Can you work these out from the model? Positions are in its coordinate system, mm. Face numbers are marked on the shaded views. A direction names the side the tool comes from. Coordinates: 2 decimals unless noted, no trailing zeros. Order: outer loops, then holes, each group sorted by start corner. A loop starts at its lowest first (then second) coordinate and runs counter-clockwise, first axis right, second up. Notation, with made-up numbers: (-36.5, 25) -> (13.5, 25) arc R36 cw to (13.5, 59) -> close; hole circle Ø1 at (12, -11). An arc over 180 degrees is marked (long way). Use a Markdown table: item, result. Add a question column.
1. If I drill on line 1 along Z through (x, y) = (-25, -5.25); line 2 along Y through (x, z) = (-4.5, 2); line 3 along X through (y, z) = (-3.25, -3.5), over which ranges is the centre line in solid material (lowest first)? Write a range as from..to.
2. Suppose I cut it at C-C, the plane y = -1.75. List the corners of the cut face in (x, z) for me, then the cut area to 3 significant figures.
3. Suppose I cut it at A-A, the plane x = -24. List the corners of the cut face in (y, z) for me, then the cut area to 3 significant figures.
4. For pin 1 Ø14 at (x, z) = (-13, -1) entering from -Y; pin 2 Ø8 at (y, z) = (-3, -1.5) entering from -X; pin 3 Ø4 at (x, z) = (-21.5, -5) entering from +Y, each with a flat end and sliding along its axis, tell me the tip position at first contact or that it passes through.
5. Suppose I cut it at B-B, the plane x = -5. List the corners of the cut face in (y, z) for me.
6. Suppose I cut it at D-D, the plane z = 14.5. List the corners of the cut face in (x, y) for me.
7. We'd pull the mould along Z, two halves only. Please class the marked faces 4, 5, 6 and 7: pulls with the +Z half, pulls with the -Z half, needs draft (parallel to the pull), parting line crosses it, or undercut.
8. For the marked faces 1, 2 and 3, which set-ups out of +Z, -Z, +X, -X, +Y, -Y let a thin tool reach every point of the face, with its end or its side?
```python
from build123d import *

# Parameters (mm, degrees)
F0_W     = 10.16
F0_H     = 5.7193874504
F1_DEPTH = 6.35
F2_DEPTH = 7.62


with BuildPart() as f1:
    # F0 (on Front) → F1 (new body, symmetric)
    with BuildSketch(Plane.XZ):
        Polygon((0, 16.9185199898), (0, 19.4585199898), (-25.4, 19.4585199898), (-25.4, 16.9185199898), (-22.86, 16.9185199898), (-12.7, 16.9185199898), (-2.54, 16.9185199898), align=None)
        with Locations((-7.62, 14.0588262645)):
            Rectangle(F0_W, F0_H)
        with Locations((-17.78, 14.0588262645)):
            Rectangle(F0_W, F0_H)
        Polygon((-3.81, 4.2185199898), (-2.54, 11.1991325393), (-12.7, 11.1991325393), (-12.7, 4.2185199898), align=None)
        Polygon((-12.7, 11.1991325393), (-22.86, 11.1991325393), (-21.59, 4.2185199898), (-12.7, 4.2185199898), align=None)
        Polygon((2.54, 4.2185199898), (-3.81, 4.2185199898), (-12.7, 4.2185199898), (-12.7, -8.4814800102), (2.54, -8.4814800102), align=None)
        Polygon((-12.7, 4.2185199898), (-21.59, 4.2185199898), (-27.94, 4.2185199898), (-27.94, -8.4814800102), (-12.7, -8.4814800102), align=None)
        Polygon((2.54, -8.4814800102), (-12.7, -8.4814800102), (-27.94, -8.4814800102), (-30.48, -8.4814800102), (-30.48, -11.0214800102), (5.0727012567, -11.0214800102), (5.08, -8.4814800102), align=None)
    extrude(amount=F1_DEPTH, both=True)

    # F0 (on Front) → F2 (join, symmetric)
    with BuildSketch(Plane.XZ):
        Polygon((0, 16.9185199898), (0, 19.4585199898), (-25.4, 19.4585199898), (-25.4, 16.9185199898), (-22.86, 16.9185199898), (-12.7, 16.9185199898), (-2.54, 16.9185199898), align=None)
    extrude(amount=F2_DEPTH, both=True)


solid = f1.part
```
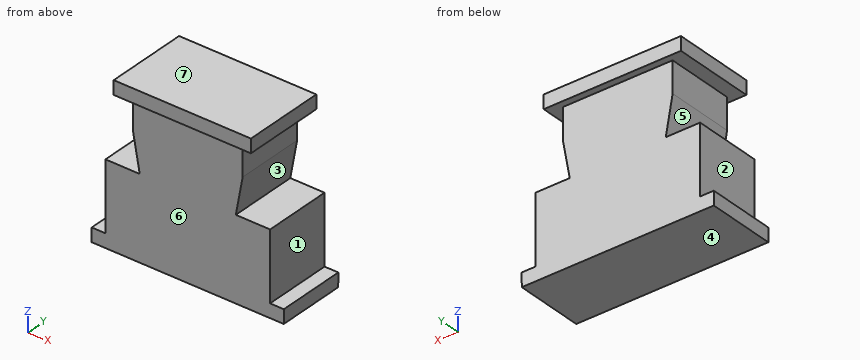
Worked out:
| question | item | result |
|---|---|---|
| 1 | line 1 | z = -11.02..4.22, 16.92..19.46 |
| 1 | line 2 | y = -6.35..6.35 |
| 1 | line 3 | x = -27.94..2.54 |
| 2 | outline | (-30.48, -11.02) -> (5.07, -11.02) -> (5.08, -8.48) -> (2.54, -8.48) -> (2.54, 4.22) -> (-3.81, 4.22) -> (-2.54, 11.2) -> (-2.54, 16.92) -> (0, 16.92) -> (0, 19.46) -> (-25.4, 19.46) -> (-25.4, 16.92) -> (-22.86, 16.92) -> (-22.86, 11.2) -> (-21.59, 4.22) -> (-27.94, 4.22) -> (-27.94, -8.48) -> (-30.48, -8.48) -> close |
| 2 | area | 791 mm² |
| 3 | outline | (-7.62, 16.92) -> (7.62, 16.92) -> (7.62, 19.46) -> (-7.62, 19.46) -> close; (-6.35, -11.02) -> (6.35, -11.02) -> (6.35, 4.22) -> (-6.35, 4.22) -> close |
| 3 | area | 232 mm² |
| 4 | pin 1 | stops at y = -6.35 |
| 4 | pin 2 | stops at x = -27.94 |
| 4 | pin 3 | stops at y = 6.35 |
| 5 | outline | (-7.62, 16.92) -> (-6.35, 16.92) -> (-6.35, -11.02) -> (6.35, -11.02) -> (6.35, 16.92) -> (7.62, 16.92) -> (7.62, 19.46) -> (-7.62, 19.46) -> close |
| 6 | outline | (-22.86, -6.35) -> (-2.54, -6.35) -> (-2.54, 6.35) -> (-22.86, 6.35) -> close |
| 7 | face 4 | pulls with the -Z half |
| 7 | face 5 | undercut |
| 7 | face 6 | needs draft |
| 7 | face 7 | pulls with the +Z half |
| 8 | face 1 | +Z, +X, +Y, -Y |
| 8 | face 2 | +Z, -X, +Y, -Y |
| 8 | face 3 | +X, +Y, -Y |
